from build123d import *

# Parameters (mm, degrees)
BOSS_EXTRUDE1_DEPTH = 2
FILLET1_R           = 1
FILLET2_R           = 1


with BuildPart() as part:
    # Sketch1 → Boss-Extrude1 (new body)
    with BuildSketch(Plane(origin=(0, 0, 0), x_dir=(1, 0, 0), z_dir=(0, 1, 0))):
        with BuildLine():
            Line((11.609772229, 3), (14.416198487, 3))
            ThreePointArc((14.416198487, 3), (9.671814624, 7.540650278), (3.127016654, 7))
            Line((3.127016654, 7), (3.127016654, 5.5))
            Line((3.127016654, 5.5), (7, 5.5))
            ThreePointArc((7, 5.5), (9.62202212, 4.834769901), (11.609772229, 3))
        make_face()
        with BuildLine():
            Line((3.127016654, -5.5), (3.127016654, -7))
            ThreePointArc((3.127016654, -7), (9.671814624, -7.540650278), (14.416198487, -3))
            Line((14.416198487, -3), (11.609772229, -3))
            ThreePointArc((11.609772229, -3), (9.62202212, -4.834769901), (7, -5.5))
            Line((7, -5.5), (3.127016654, -5.5))
        make_face()
        with BuildLine():
            Line((3.127016654, -5.5), (1.190524981, -5.5))
            ThreePointArc((1.190524981, -5.5), (2.101020514, -6.32455532), (3.127016654, -7))
            Line((3.127016654, -7), (3.127016654, -5.5))
        make_face()
        with BuildLine():
            ThreePointArc((0, -3.872983346), (0.543804652, -4.72414454), (1.190524981, -5.5))
            Line((1.190524981, -5.5), (3.127016654, -5.5))
            Line((3.127016654, -5.5), (3.127016654, -3.905124838))
            ThreePointArc((3.127016654, -3.905124838), (2.734545947, -3.472160958), (2.390227771, -3))
            Line((2.390227771, -3), (0.416198487, -3))
            ThreePointArc((0.416198487, -3), (0.221303185, -3.442786708), (0, -3.872983346))
        make_face()
        with BuildLine():
            ThreePointArc((1, 0), (0.85269342, -1.5281381), (0.416198487, -3))
            Line((0.416198487, -3), (2.390227771, -3))
            ThreePointArc((2.390227771, -3), (1.5, 0), (2.390227771, 3))
            Line((2.390227771, 3), (0.416198487, 3))
            ThreePointArc((0.416198487, 3), (0.85269342, 1.5281381), (1, 0))
        make_face()
        with BuildLine():
            ThreePointArc((0, 3.872983346), (0.221303185, 3.442786708), (0.416198487, 3))
            Line((0.416198487, 3), (2.390227771, 3))
            ThreePointArc((2.390227771, 3), (2.734545947, 3.472160958), (3.127016654, 3.905124838))
            Line((3.127016654, 3.905124838), (3.127016654, 5.5))
            Line((3.127016654, 5.5), (1.190524981, 5.5))
            ThreePointArc((1.190524981, 5.5), (0.543804652, 4.72414454), (0, 3.872983346))
        make_face()
        with BuildLine():
            Line((1.190524981, 5.5), (-1.190524981, 5.5))
            ThreePointArc((-1.190524981, 5.5), (-0.543804652, 4.72414454), (0, 3.872983346))
            ThreePointArc((0, 3.872983346), (0.543804652, 4.72414454), (1.190524981, 5.5))
        make_face()
        with BuildLine():
            Line((-1.190524981, 5.5), (-3.127016654, 5.5))
            Line((-3.127016654, 5.5), (-3.127016654, 3.905124838))
            ThreePointArc((-3.127016654, 3.905124838), (-2.734545947, 3.472160958), (-2.390227771, 3))
            Line((-2.390227771, 3), (-0.416198487, 3))
            ThreePointArc((-0.416198487, 3), (-0.221303185, 3.442786708), (0, 3.872983346))
            ThreePointArc((0, 3.872983346), (-0.543804652, 4.72414454), (-1.190524981, 5.5))
        make_face()
        with BuildLine():
            ThreePointArc((-1.5, 0), (-1.727251795, -1.564648961), (-2.390227771, -3))
            Line((-2.390227771, -3), (-0.416198487, -3))
            ThreePointArc((-0.416198487, -3), (-1, 0), (-0.416198487, 3))
            Line((-0.416198487, 3), (-2.390227771, 3))
            ThreePointArc((-2.390227771, 3), (-1.727251795, 1.564648961), (-1.5, 0))
        make_face()
        with BuildLine():
            Line((-3.127016654, -3.905124838), (-3.127016654, -5.5))
            Line((-3.127016654, -5.5), (-1.190524981, -5.5))
            ThreePointArc((-1.190524981, -5.5), (-0.543804652, -4.72414454), (0, -3.872983346))
            ThreePointArc((0, -3.872983346), (-0.221303185, -3.442786708), (-0.416198487, -3))
            Line((-0.416198487, -3), (-2.390227771, -3))
            ThreePointArc((-2.390227771, -3), (-2.734545947, -3.472160958), (-3.127016654, -3.905124838))
        make_face()
        with BuildLine():
            ThreePointArc((0, -3.872983346), (-0.543804652, -4.72414454), (-1.190524981, -5.5))
            Line((-1.190524981, -5.5), (1.190524981, -5.5))
            ThreePointArc((1.190524981, -5.5), (0.543804652, -4.72414454), (0, -3.872983346))
        make_face()
        with BuildLine():
            ThreePointArc((-0.416198487, 3), (-1, 0), (-0.416198487, -3))
            Line((-0.416198487, -3), (0.416198487, -3))
            ThreePointArc((0.416198487, -3), (0.85269342, -1.5281381), (1, 0))
            ThreePointArc((1, 0), (0.85269342, 1.5281381), (0.416198487, 3))
            Line((0.416198487, 3), (-0.416198487, 3))
        make_face()
        with BuildLine():
            ThreePointArc((0, 3.872983346), (-0.221303185, 3.442786708), (-0.416198487, 3))
            Line((-0.416198487, 3), (0.416198487, 3))
            ThreePointArc((0.416198487, 3), (0.221303185, 3.442786708), (0, 3.872983346))
        make_face()
        with BuildLine():
            ThreePointArc((-0.416198487, -3), (-0.221303185, -3.442786708), (0, -3.872983346))
            ThreePointArc((0, -3.872983346), (0.221303185, -3.442786708), (0.416198487, -3))
            Line((0.416198487, -3), (-0.416198487, -3))
        make_face()
        with BuildLine():
            Line((-3.127016654, 5.5), (-7, 5.5))
            ThreePointArc((-7, 5.5), (-4.905744358, 5.085675305), (-3.127016654, 3.905124838))
            Line((-3.127016654, 3.905124838), (-3.127016654, 5.5))
        make_face()
        with BuildLine():
            Line((-14.416198487, 3), (-11.609772229, 3))
            ThreePointArc((-11.609772229, 3), (-9.62202212, 4.834769901), (-7, 5.5))
            Line((-7, 5.5), (-3.127016654, 5.5))
            Line((-3.127016654, 5.5), (-3.127016654, 7))
            ThreePointArc((-3.127016654, 7), (-9.671814624, 7.540650278), (-14.416198487, 3))
        make_face()
        with BuildLine():
            Line((-3.127016654, 7), (-3.127016654, 5.5))
            Line((-3.127016654, 5.5), (-1.190524981, 5.5))
            ThreePointArc((-1.190524981, 5.5), (-2.101020514, 6.32455532), (-3.127016654, 7))
        make_face()
        with BuildLine():
            Line((3.127016654, 5.5), (3.127016654, 7))
            ThreePointArc((3.127016654, 7), (2.101020514, 6.32455532), (1.190524981, 5.5))
            Line((1.190524981, 5.5), (3.127016654, 5.5))
        make_face()
        with BuildLine():
            Line((-1.190524981, -5.5), (-3.127016654, -5.5))
            Line((-3.127016654, -5.5), (-3.127016654, -7))
            ThreePointArc((-3.127016654, -7), (-2.101020514, -6.32455532), (-1.190524981, -5.5))
        make_face()
        with BuildLine():
            Line((-3.127016654, -5.5), (-7, -5.5))
            ThreePointArc((-7, -5.5), (-9.62202212, -4.834769901), (-11.609772229, -3))
            Line((-11.609772229, -3), (-14.416198487, -3))
            ThreePointArc((-14.416198487, -3), (-9.671814624, -7.540650278), (-3.127016654, -7))
            Line((-3.127016654, -7), (-3.127016654, -5.5))
        make_face()
        with BuildLine():
            ThreePointArc((-3.127016654, -3.905124838), (-4.905744358, -5.085675305), (-7, -5.5))
            Line((-7, -5.5), (-3.127016654, -5.5))
            Line((-3.127016654, -5.5), (-3.127016654, -3.905124838))
        make_face()
        with BuildLine():
            Line((7, 5.5), (3.127016654, 5.5))
            Line((3.127016654, 5.5), (3.127016654, 3.905124838))
            ThreePointArc((3.127016654, 3.905124838), (4.905744358, 5.085675305), (7, 5.5))
        make_face()
        with BuildLine():
            Line((3.127016654, -3.905124838), (3.127016654, -5.5))
            Line((3.127016654, -5.5), (7, -5.5))
            ThreePointArc((7, -5.5), (4.905744358, -5.085675305), (3.127016654, -3.905124838))
        make_face()
    extrude(amount=BOSS_EXTRUDE1_DEPTH)

    # Fillet1
    fillet1_edges = [part.edges().sort_by_distance(p)[0] for p in [
        (-14.416198487, 1, -3),
        (14.416198487, 1, -3),
        (14.416198487, 1, 3),
        (-14.416198487, 1, 3),
    ]]
    fillet(fillet1_edges, radius=FILLET1_R)

    # Fillet2
    fillet2_edges = [part.edges().sort_by_distance(p)[0] for p in [
        (-11.609772229, 1, 3),
        (-11.609772229, 1, -3),
        (11.609772229, 1, -3),
        (11.609772229, 1, 3),
    ]]
    fillet(fillet2_edges, radius=FILLET2_R)


solid = part.part
Model file for the job. Use its own axes, mm. A direction names the side the tool comes from. Coordinates: 2 decimals unless noted, no trailing zeros. Write each loop counter-clockwise with the first axis right and the second up, starting at its lowest first coordinate (ties: lowest second). Pieces come first, ordered by that corner, then holes. Notation, with made-up numbers: (15, 78) -> (27, 78) arc R31 ccw to (27, 116) -> close; hole circle Ø8 at (89.5, 82). An arc over 180 degrees is marked (long way). One line per item, written item: value. Start each with the question number.
1) Pull direction Z, two halves, no side cores. Call faces 1 (the face through (0, 0, 0)), 2 (the face through (-13.638, 1.014, -3.551)), 3 (the face through (0, 1, -5.5)): +Z half, -Z half, draft (parallel to the pull), parting line (faces both ways), or undercut.
2) Slice it at D-D on z = -1. Write the cut outline in (x, y), then the cut area to 3 significant figures.
3) Flat gauge pins, fed straight in: pin 1 Ø1 at (x, y) = (0, 1) entering from -Z; pin 2 Ø1 at (x, z) = (-4, -6.5) entering from -Y; pin 3 Ø0.7 at (x, y) = (-12.5, 0.5) entering from -Z; pin 4 Ø2 at (x, z) = (-10, 2.5) entering from +Y. Where does each tip first touch, or does it go through?
4) Probe probe 1 along X at (y, z) = (0.85, -3.75); probe 2 along X at (y, z) = (0.45, -4); probe 3 along Z at (x, y) = (-1, 1.2). List the from-to ranges inside material, lowest first.
5) Slice it at C-C on x = -7.5. Write the cut outline in (y, z).
6) Which spindle directions (+Z, -Z, +X, -X, +Y, -Y) get a long thin tool onto all of the face, cutting with end or side? Do faces 4 (the face through (0, 1, 5.5)), 5 (the face through (13.62, 1.01, -3.52)). Say none if no direction does.
7) Slice it at B-B on z = -5. Write the cut outline in (x, y) (3 decimals).
8) Slice it at A-A on x = -3.5. Write the cut outline in (y, z), then the cut area to 3 significant figures.
Answers follow:
1. face 1: draft
1. face 2: undercut
1. face 3: -Z half
2. outline: (-1.59, 0) -> (1.59, 0) -> (1.59, 2) -> (-1.59, 2) -> close
2. area: 6.37 mm2
3. pin 1: z = -5.5
3. pin 2: y = 0
3. pin 3: z = -6.12
3. pin 4: through
4. probe 1: -13.71 to -11.02, -2.98 to 2.98, 11.02 to 13.71
4. probe 2: -13.74 to -10.77, -3.23 to 3.23, 10.77 to 13.74
4. probe 3: -5.5 to 5.5
5. outline: (0, -7.98) -> (2, -7.98) -> (2, -5.48) -> (0, -5.48) -> close; (0, 5.48) -> (2, 5.48) -> (2, 7.98) -> (0, 7.98) -> close
6. face 4: +Z, +Y, -Y
6. face 5: +X, +Y, -Y
7. outline: (-13.245, 0) -> (-9.291, 0) -> (-9.291, 2) -> (-13.245, 2) -> close; (-4.709, 0) -> (4.709, 0) -> (4.709, 2) -> (-4.709, 2) -> close; (9.291, 0) -> (13.245, 0) -> (13.245, 2) -> (9.291, 2) -> close
8. outline: (0, -7.19) -> (2, -7.19) -> (2, -4.24) -> (0, -4.24) -> close; (0, 4.24) -> (2, 4.24) -> (2, 7.19) -> (0, 7.19) -> close
8. area: 11.8 mm2
